Could you check a few things on this drawing? It's one solid part, dimensions in mm from its lowest x, y, z. A direction names the side the tool comes from. Give positions to 0.01 mm unless a question says otherwise; leave off trailing zeros. Loops run counter-clockwise (first coordinate to the right, second up) from the corner with the lowest first, then second, coordinate; pieces in that order, holes last.
Q1. Suppose I cut it at B-B (z = 2.5). List the corners of the cut face in (x, y) for me.
Q2. For the marked faces 1 and 2, which set-ups out of +Z, -Z, +X, -X, +Y, -Y let a thin tool reach every point of the face, with its end or its side?
Q3. Thinking about a two-plate mould opening in X: for the marked faces 3, 4 and 5, which applies, pulls with the +X half, pulls with the -X half, needs draft (parallel to the pull), parting line crosses it, or undercut?
Q4. I'm going to push flat-ended pins straight in: P1, Ø1, axis at x = 31, y = 29.5, coming from the +Z side; P2, Ø1.5, axis at x = 15.5, z = 14.5, coming from the -Y side; P3, Ø5, axis at x = 22.5, z = 16.5, coming from the +Y side; P4, Ø3, axis at x = 17.5, y = 38, coming from the +Z side. Where does each tip first touch, or does it pass through?
Q5. Suppose I cut it at A-A (y = 22.5). List the corners of the cut face in (x, z) for me.
Q6. I need wall thicknesses on probe 1 along Z at (x, y) = (23, 6.5); probe 2 along Y at (x, z) = (30.5, 8.5); probe 3 along X at (y, z) = (21.25, 15). Which ranges of each line are inside material? Lowest first, please.
Q7. Suppose I cut it at C-C (z = 15.75). List the corners of the cut face in (x, y) for me.
Q8. Suppose I cut it at D-D (y = 38). List the corners of the cut face in (x, z) for me.
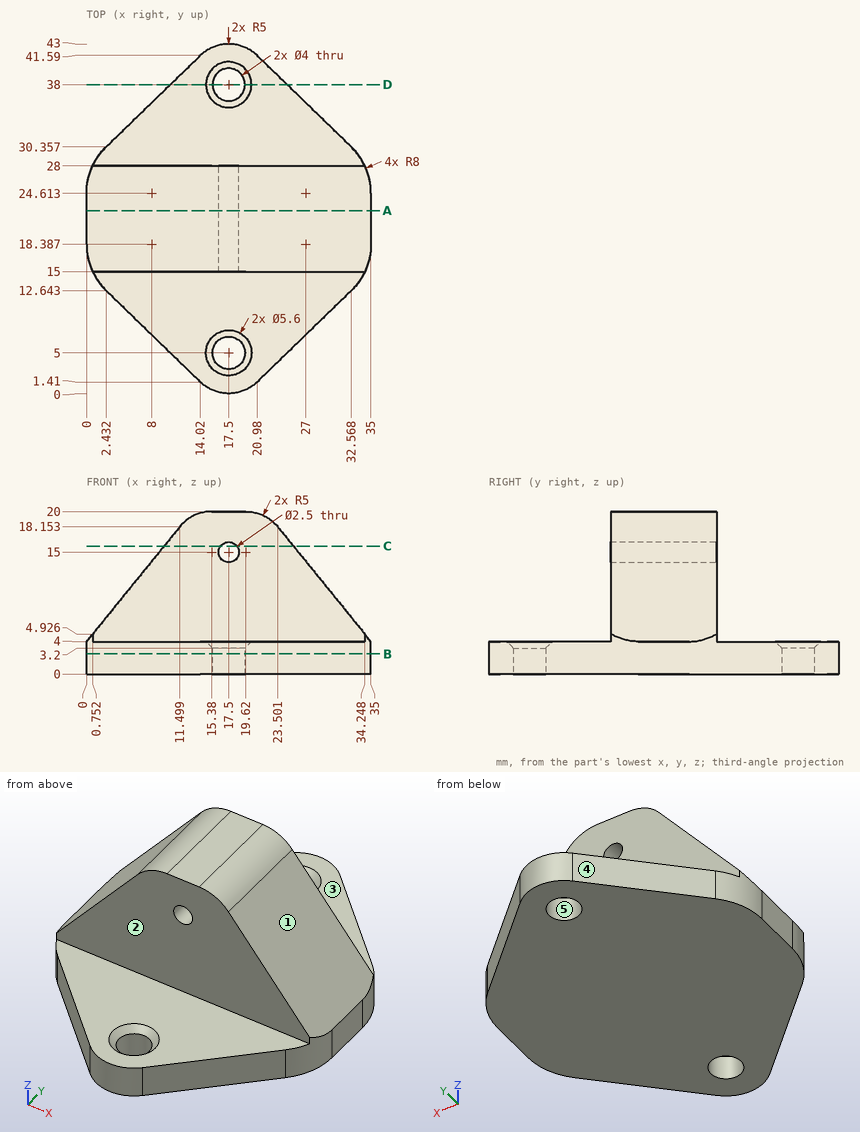
Solutions:
1. outline: (0, 18.39) arc R8 ccw to (2.43, 12.64) - (14.02, 1.41) arc R5 ccw to (20.98, 1.41) - (32.57, 12.64) arc R8 ccw to (35, 18.39) - (35, 24.61) arc R8 ccw to (32.57, 30.36) - (20.98, 41.59) arc R5 ccw to (14.02, 41.59) - (2.43, 30.36) arc R8 ccw to (0, 24.61) - close; hole circle Ø4 at (17.5, 5); hole circle Ø4 at (17.5, 38)
2. face 1: +Z, +X, +Y, -Y
2. face 2: +Z, +X, -X, -Y
3. face 3: needs draft
3. face 4: pulls with the -X half
3. face 5: undercut
4. P1: stops at z = 4
4. P2: stops at y = 15
4. P3: stops at y = 28
4. P4: passes through
5. outline: (0, 0) - (35, 0) - (35, 4) - (23.5, 18.15) arc R5 ccw to (19.62, 20) - (15.38, 20) arc R5 ccw to (11.5, 18.15) - (0, 4) - close; hole circle Ø2.5 at (17.5, 15)
6. probe 1: z = 0 to 4
6. probe 2: y = 15 to 28
6. probe 3: x = 8.94 to 16.25, 18.75 to 26.06
7. outline: (9.55, 15) - (16.5, 15) - (16.5, 28) - (9.55, 28) - close; (18.5, 15) - (25.45, 15) - (25.45, 28) - (18.5, 28) - close
8. outline: (10.32, 0) - (15.5, 0) - (15.5, 3.2) - (14.7, 4) - (10.32, 4) - close; (19.5, 0) - (24.68, 0) - (24.68, 4) - (20.3, 4) - (19.5, 3.2) - close
